Check sheet for the drawn part. Datum: minimum x, y, z corner. Units: mm. A direction names the side the tool comes from. Coordinates: 2 decimals unless noted, no trailing zeros. Write each loop counter-clockwise with the first axis right and the second up, starting at its lowest first coordinate (ties: lowest second). Pieces come first, ordered by that corner, then holes. Notation, with made-up numbers: (83, -35) -> (95, -35) arc R32 ccw to (95, -4) -> close; hole circle Ø8 at (48.25, -18.75). An arc over 180 degrees is marked (long way). Answer in a Markdown table with one row per item. Add a question column.
1. Cross-section at B-B on z = 29. Record the cut outline in (x, y).
2. Cross-section at D-D on x = 85. Record the cut outline in (y, z).
3. Scan lines: L1, parallel to Z at x = 88.5, y = 32; L2, parallel to Y at x = 98, z = 24; L3, parallel to X at y = 48.5, z = 18. Record each from-to range of solid material in increasing order. Write a range as from..to.
4. Cross-section at C-C on x = 125. Record the cut outline in (y, z), and give its area (3 significant figures).
5. Set-up check for the marked faces 1 and 2: record each of +Z, -Z, +X, -X, +Y, -Y from which the full face is reachable in a straight line by a thin tool's end or side.
6. Cross-section at A-A on y = 16. Record the cut outline in (x, z), and give its area (3 significant figures).
7. Mould release check, pull along Z, two halves, no side actions. Record for the marked faces 3, 4 and 5: pulls with the +Z half, pulls with the -Z half, needs draft (parallel to the pull), parting line crosses it, or undercut.
8. Depth check by flat-ended pin: P1, Ø12, axis at x = 122.5, z = 12, coming from the -Y side. Enter the tip coordinate at first touch or a pass-through.
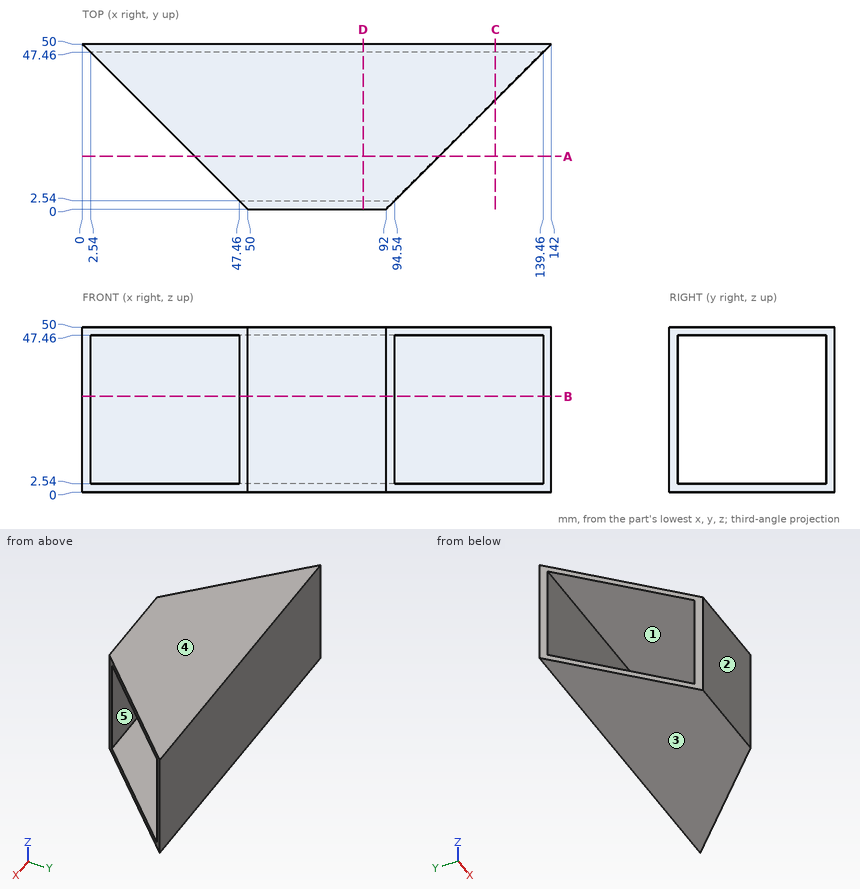
Results found:
| question | item | result |
|---|---|---|
| 1 | outline | (0, 50) -> (2.54, 47.46) -> (139.46, 47.46) -> (142, 50) -> close; (47.46, 2.54) -> (50, 0) -> (92, 0) -> (94.54, 2.54) -> close |
| 2 | outline | (0, 0) -> (50, 0) -> (50, 50) -> (0, 50) -> close; hole (2.54, 2.54) -> (47.46, 2.54) -> (47.46, 47.46) -> (2.54, 47.46) -> close |
| 3 | L1 | z = 0..2.54, 47.46..50 |
| 3 | L2 | y = 47.46..50 |
| 3 | L3 | x = 1.5..140.5 |
| 4 | outline | (33, 0) -> (50, 0) -> (50, 50) -> (33, 50) -> (33, 47.46) -> (47.46, 47.46) -> (47.46, 2.54) -> (33, 2.54) -> close |
| 4 | area | 200 mm^2 |
| 5 | face 1 | +X, -X |
| 5 | face 2 | +Z, -Z, +X, -X, -Y |
| 6 | outline | (34, 0) -> (108, 0) -> (108, 2.54) -> (34, 2.54) -> close; (34, 47.46) -> (108, 47.46) -> (108, 50) -> (34, 50) -> close |
| 6 | area | 376 mm^2 |
| 7 | face 3 | pulls with the -Z half |
| 7 | face 4 | pulls with the +Z half |
| 7 | face 5 | undercut |
| 8 | P1 | stops at y = 47.46 |
